from build123d import *

# Parameters (mm, degrees)
F1_DEPTH = 19.05
F2_R     = 6.35
F4_D     = 9.525


with BuildPart() as f1:
    # F0 (on Front) → F1 (new body)
    with BuildSketch(Plane.XZ):
        Polygon((-11.738134, 16.807301), (-30.788134, 16.807301), (-30.788134, 4.107301), (0.961866, 4.107301), (0.961866, 29.507301), (-11.738134, 29.507301), align=None)
    extrude(amount=F1_DEPTH)

    # F2
    f2_edges = [f1.edges().sort_by_distance(p)[0] for p in [
        (-30.788134, 0, 10.457301),
        (-30.788134, -19.05, 10.457301),
        (-11.738134, -9.525, 16.807301),
    ]]
    fillet(f2_edges, radius=F2_R)

    # F4 (through all)
    with Locations(Plane.XY.offset(16.807301)):
        with Locations((-23.808645, -10.041741)):
            Hole(F4_D / 2)

    # F5: F1 across plane


with BuildPart() as f1_1:
    add(f1.part)
    add(f1.part.mirror(Plane.YZ))


solid = f1_1.part
Check sheet for the modelled part. Datum: model origin and axes. Units: mm. A direction names the side the tool comes from. Round coordinates to 2 decimals unless told otherwise and drop trailing zeros. Loops run counter-clockwise (first coordinate to the right, second up) from the corner with the lowest first, then second, coordinate; pieces in that order, holes last. Notation, with made-up numbers: M 68.25,40.5 L 102.25,40.5 A15 cw 102.25,59.5 Z; hole C 75.25,3 d2. An arc over 180 degrees is marked long. One line per question, with ' | ' between items. Start each with the question number.
Item 1: Section check A-A (y = -11.25). Record the boundary of the cut face in (x, z), and give its area (3 significant figures).
Item 2: Scan lines: probe 1 along X at (y, z) = (-10, 5.5); probe 2 along X at (y, z) = (-7.75, 6.75); probe 3 along Z at (x, y) = (23, -3.75). Record each from-to range of solid material in increasing order.
Item 3: Release check for a two-part mould opening along X. For faces 4 (the face through (-13.648, -9.658, 18.618)), 5 (the face through (0, -9, 29.507)), 6 (the face through (28.35, -8.61, 10.37)) record: released by +X, released by -X, zero draft, split by the parting line, or undercut.
Item 4: Section check C-C (z = 6.75). State how many separate pieces and enclosed holes the cut face has, and give its area (3 significant figures).
Item 5: Section check D-D (y = -2.25). Record the boundary of the cut face in (x, z), and give its area (3 significant figures).
Item 6: Set-up check for faces 1 (the face through (11.738, -9, 26)), 2 (the face through (-30.788, -9, 11)), 3 (the face through (-11.738, -9, 26)): record each of +Z, -Z, +X, -X, +Y, -Y from which the full face is reachable in a straight line by a thin tool's end or side.
Item 7: Section check B-B (x = 23). Record the boundary of the cut face in (y, z).
Item 8: Gauge pin test, flat ends, axial feed: pin 1 Ø4 at (x, y) = (-21.5, -7.5) entering from +Z; pin 2 Ø7 at (y, z) = (-13, 25.5) entering from +X; pin 3 Ø5 at (y, z) = (-13.5, 28) entering from -X. Record the tip position at first contact, or that the pin passes through.
Worked out:
1) outline: M -30.79,4.11 L -28.42,4.11 L -28.42,16.81 L -30.79,16.81 Z; M -19.2,4.11 L 19.2,4.11 L 19.2,16.81 L 18.09,16.81 A6.35 cw 11.74,23.16 L 11.74,29.51 L -11.74,29.51 L -11.74,23.16 A6.35 cw -18.09,16.81 L -19.2,16.81 Z; M 28.42,4.11 L 30.79,4.11 L 30.79,16.81 L 28.42,16.81 Z | area: 863 mm^2
2) probe 1: -30.79 to -28.57, -19.05 to 19.05, 28.57 to 30.79 | probe 2: -30.79 to -27.98, -19.63 to 19.63, 27.98 to 30.79 | probe 3: 4.11 to 16.81
3) face 4: released by -X | face 5: zero draft | face 6: undercut
4) separate pieces: 1 | enclosed holes: 2 | area: 996 mm^2
5) outline: M -29.29,4.11 L 29.29,4.11 L 29.29,16.81 L 18.09,16.81 A6.35 cw 11.74,23.16 L 11.74,29.51 L -11.74,29.51 L -11.74,23.16 A6.35 cw -18.09,16.81 L -29.29,16.81 Z | area: 1,060 mm^2
6) face 1: +Z, +X, +Y, -Y | face 2: +Z, -Z, -X, +Y, -Y | face 3: +Z, -X, +Y, -Y
7) outline: M -19.05,4.11 L -14.74,4.11 L -14.74,16.81 L -19.05,16.81 Z; M -5.35,4.11 L 0,4.11 L 0,16.81 L -5.35,16.81 Z
8) pin 1: z = 16.81 | pin 2: x = 11.84 | pin 3: x = -11.74
